Model file for the job. Use its own axes, mm. Round coordinates to 2 decimals unless told otherwise and drop trailing zeros. Order: outer loops, then holes, each group sorted by start corner. A loop starts at its lowest first (then second) coordinate and runs counter-clockwise, first axis right, second up. Notation, with made-up numbers: (-15.75, -29) -> (14.25, -29) arc R20 cw to (14.25, 7) -> close; hole circle Ø11 at (-6.5, 75). An arc over 180 degrees is marked (long way). Put each result on its own line as item: value. Start each with the question number.
Q1. Probe L1, parallel to X at y = -0.5, z = 3; L2, parallel to X at y = 1.5, z = 0.75; L3, parallel to Y at x = -237, z = 4. List the from-to ranges inside material, lowest first.
Q2. Cut at C-C, the plane z = 1. List the corners of the cut face in (x, y) (1 decimal).
Q3. Cut at B-B, the plane y = 4. List the corners of the cut face in (x, z), and give its area (3 significant figures).
Q4. Flat gauge pins, fed straight in: P1, Ø3, axis at y = 61, z = 3, coming from the +X side; P2, Ø2, axis at y = -0.5, z = 5, coming from the -X side; P3, Ø3, axis at y = 58, z = 3, coming from the -X side. Where does each tip first touch, or does it go through?
Q5. Cut at D-D, the plane x = -189. List the corners of the cut face in (y, z).
Q6. Cut at A-A, the plane y = 60. List the corners of the cut face in (x, z).
from build123d import *

# Parameters (mm, degrees)
SKETCH1_R           = 14.2875
SKETCH1_R_2         = 9.398
BOSS_EXTRUDE1_DEPTH = 6.35
FILLET1_R           = 20.32
FILLET4_R           = 20.32
FILLET5_R           = 20.32
FILLET6_R           = 20.32


with BuildPart() as part:
    # Sketch1 → Boss-Extrude1 (new body)
    with BuildSketch(Plane.XY):
        with BuildLine():
            Line((0, -24.13), (-313.436, -24.13))
            ThreePointArc((-313.436, -24.13), (-337.49260416, -0.07339584), (-313.436, 23.98320832))
            Line((-313.436, 23.98320832), (-90.24339584, 23.98320832))
            Line((-90.24339584, 23.98320832), (-90.24339584, 88.82660416))
            Line((-90.24339584, 88.82660416), (-25.286322176, 88.82660416))
            Line((-25.286322176, 88.82660416), (-25.286322176, 23.98320832))
            Line((-25.286322176, 23.98320832), (0, 24.13))
            ThreePointArc((0, 24.13), (24.13, 0), (0, -24.13))
        make_face()
        with Locations((-313.436, -0.07339584)):
            Circle(SKETCH1_R, mode=Mode.SUBTRACT)
        Circle(SKETCH1_R, mode=Mode.SUBTRACT)
        with Locations((-57.764858946, 56.47830208)):
            Circle(SKETCH1_R_2, mode=Mode.SUBTRACT)
    extrude(amount=BOSS_EXTRUDE1_DEPTH)

    # Fillet1
    fillet1_edges = [part.edges().sort_by_distance(p)[0] for p in [
        (-90.24339584, 23.98320832, 3.175),
    ]]
    fillet(fillet1_edges, radius=FILLET1_R)

    # Fillet4
    fillet4_edges = [part.edges().sort_by_distance(p)[0] for p in [
        (-25.286322176, 23.98320832, 3.175),
    ]]
    fillet(fillet4_edges, radius=FILLET4_R)

    # Fillet5
    fillet5_edges = [part.edges().sort_by_distance(p)[0] for p in [
        (-25.286322176, 88.82660416, 3.175),
    ]]
    fillet(fillet5_edges, radius=FILLET5_R)

    # Fillet6
    fillet6_edges = [part.edges().sort_by_distance(p)[0] for p in [
        (-90.24339584, 88.82660416, 3.175),
    ]]
    fillet(fillet6_edges, radius=FILLET6_R)


solid = part.part
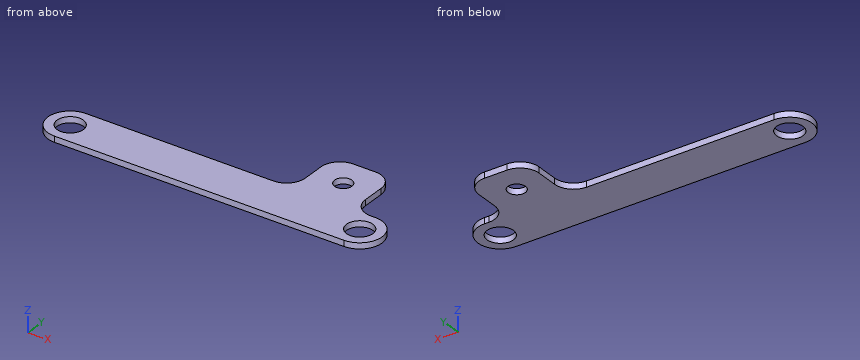
Ans:
1. L1: x = -337.49 to -327.72, -299.15 to -14.28, 14.28 to 24.12
1. L2: x = -337.44 to -327.64, -299.24 to -14.21, 14.21 to 24.08
1. L3: y = -24.13 to 23.98
2. outline: (-313.4, -24.1) -> (0, -24.1) arc R24.1 ccw to (0, 24.1) -> (-4.8, 24.1) arc R20.3 cw to (-25.3, 44.4) -> (-25.3, 68.5) arc R20.3 ccw to (-45.6, 88.8) -> (-69.9, 88.8) arc R20.3 ccw to (-90.2, 68.5) -> (-90.2, 44.3) arc R20.3 cw to (-110.6, 24) -> (-313.4, 24) arc R24.1 ccw to start; hole circle Ø28.6 at (-313.4, -0.1); hole circle Ø18.8 at (-57.8, 56.5); hole circle Ø28.6 at (0, 0)
3. outline: (-337.15, 0) -> (-327.13, 0) -> (-327.13, 6.35) -> (-337.15, 6.35) -> close; (-299.74, 0) -> (-13.72, 0) -> (-13.72, 6.35) -> (-299.74, 6.35) -> close; (13.72, 0) -> (23.8, 0) -> (23.8, 6.35) -> (13.72, 6.35) -> close
3. area: 1,940 mm^2
4. P1: stops at x = -25.29
4. P2: stops at x = -337.49
4. P3: stops at x = -90.24
5. outline: (-24.13, 0) -> (23.98, 0) -> (23.98, 6.35) -> (-24.13, 6.35) -> close
6. outline: (-90.24, 0) -> (-66.48, 0) -> (-66.48, 6.35) -> (-90.24, 6.35) -> close; (-49.05, 0) -> (-25.29, 0) -> (-25.29, 6.35) -> (-49.05, 6.35) -> close
